Verification items for this drawing (mm, ordinates from the low corner). A direction names the side the tool comes from. Round coordinates to 2 decimals unless told otherwise and drop trailing zeros. Order: outer loops, then holes, each group sorted by start corner. A loop starts at its lowest first (then second) coordinate and runs counter-clockwise, first axis right, second up. Notation, with made-up numbers: (41, 3) -> (74, 3) arc R28 cw to (74, 21) -> close; hole circle Ø1 at (-22.5, -16.75). An arc over 180 degrees is marked (long way). Return JSON: item names as keys, results as strings. Group by question number.
Item 1: Scan lines: probe 1 along Z at (x, y) = (15.5, 6); probe 2 along Z at (x, y) = (11.5, 4.5); probe 3 along Y at (x, z) = (29.5, 7). Record each from-to range of solid material in increasing order. Write a range as from..to.
Item 2: Sectioned sample at A-A on z = 15. Record the cut outline in (x, y).
Item 3: Draft check along X on the marked faces 3, 4 and 5. Enter one of: pulls with the +X half, pulls with the -X half, needs draft (parallel to the pull), parting line crosses it, or undercut.
Item 4: Depth check by flat-ended pin: pin 1 Ø2 at (y, z) = (4, 27) entering from +X (1 decimal); pin 2 Ø1.5 at (x, y) = (10, 5) entering from +Z (1 decimal); pin 3 Ø1.5 at (x, y) = (8.5, 2) entering from -Z. Enter the tip coordinate at first touch or a pass-through.
Item 5: Access from +Z, -Z, +X, -X, +Y, -Y to the whole of each face (thin tool, end or side, straight path). Record for the marked faces 1 and 2.
Item 6: Sectioned sample at C-C on z = 32. Record the cut outline in (x, y), plus the area to 3 significant figures.
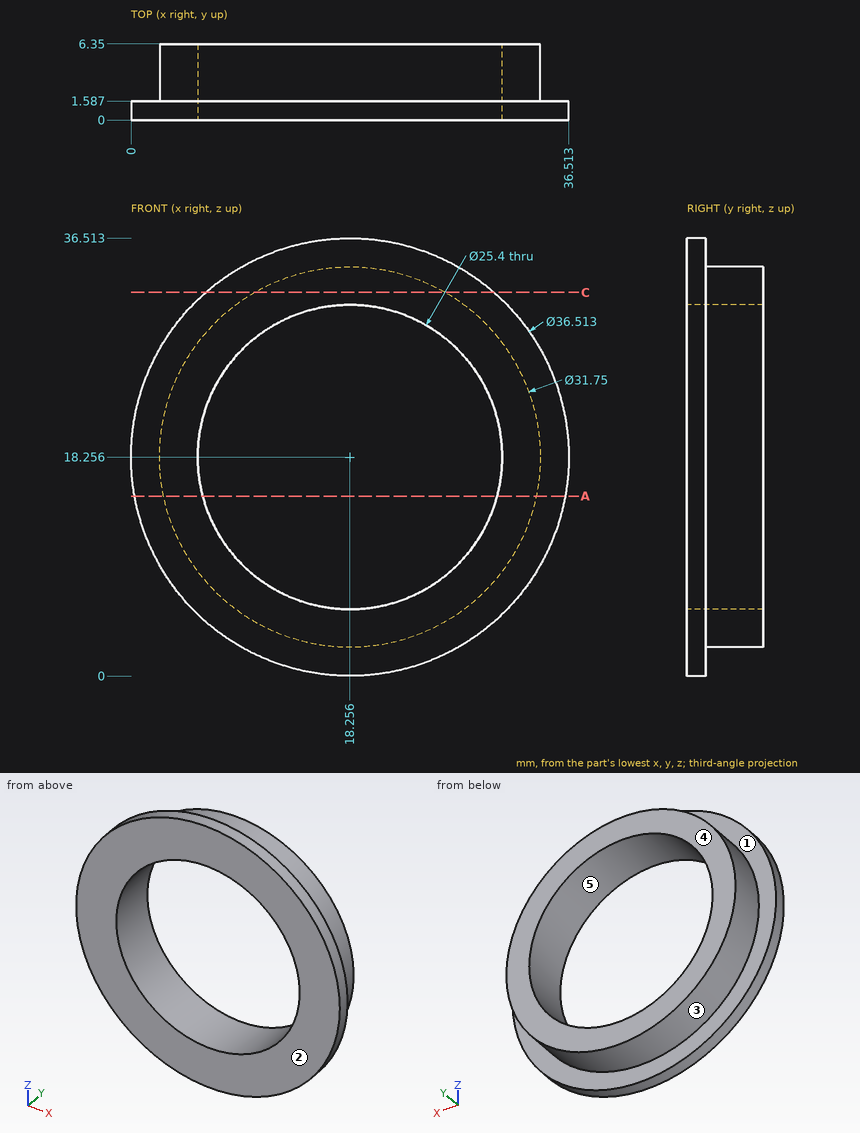
Recorded:
{
 "1": {"probe 1": "2.62..5.86, 30.65..33.89", "probe 2": "3.89..7.5, 29.01..32.62", "probe 3": "0..1.59"},
 "2": {"outline": "(0.29, 0) -> (5.98, 0) -> (5.98, 6.35) -> (2.72, 6.35) -> (2.72, 1.59) -> (0.29, 1.59) -> close; (30.53, 0) -> (36.22, 0) -> (36.22, 1.59) -> (33.79, 1.59) -> (33.79, 6.35) -> (30.53, 6.35) -> close"},
 "3": {"face 3": "parting line crosses it", "face 4": "needs draft", "face 5": "undercut"},
 "4": {"pin 1": "x = 32.1", "pin 2": "z = 32.2", "pin 3": "z = 2.45"},
 "5": {"face 1": "+Y", "face 2": "+Z, -Z, +X, -X, -Y"},
 "6": {"outline": "(6.24, 0) -> (30.27, 0) -> (30.27, 1.59) -> (26.2, 1.59) -> (26.2, 6.35) -> (10.31, 6.35) -> (10.31, 1.59) -> (6.24, 1.59) -> close", "area": "114 mm²"}
}
